Model file for the job. Use its own axes, mm. A direction names the side the tool comes from. Round coordinates to 2 decimals unless told otherwise and drop trailing zeros. Order: outer loops, then holes, each group sorted by start corner. A loop starts at its lowest first (then second) coordinate and runs counter-clockwise, first axis right, second up. Notation, with made-up numbers: (47.25, 61) - (87.25, 61) arc R11 cw to (87.25, 73) - close; hole circle Ø5 at (37, -26). An arc over 180 degrees is marked (long way). Put each result on its own line as item: value. Start each with the question number.
Item 1: Saw through at D-D on x = 8.5. List the corners of the cut face in (y, z), plus the area to 3 significant figures.
Item 2: Saw through at A-A on z = 9.25. List the corners of the cut face in (x, y).
Item 3: Saw through at C-C on z = -2. List the corners of the cut face in (x, y).
Item 4: Mould opens along X. For faces 4 (the face through (-11, 0, 1)), 5 (the face through (4, 0, 11.15)), 6 (the face through (0, 3, 2)) say: pulls with the +X half, pulls with the -X half, needs draft (parallel to the pull), parting line crosses it, or undercut.
Item 5: Saw through at B-B on y = -0.7. State how many separate pieces and enclosed holes the cut face has, plus the area to 3 significant figures.
Item 6: Which spindle directions (+Z, -Z, +X, -X, +Y, -Y) get a long thin tool onto all of the face, cutting with end or side? Do faces 1 (the face through (-6.1, 0, 7)), 2 (the face through (-1.984, 1, 7)), 3 (the face through (6.1, 0, 7)). Say none if no direction does.
Item 7: Probe probe 1 along X at (y, z) = (-1.5, 4.5); probe 2 along X at (y, z) = (1.3, -7.75); probe 3 along Z at (x, y) = (4, 1.45). List the from-to ranges inside material, lowest first.
Item 8: Pin check, flat tips, straight feed: pin 1 Ø3 at (x, y) = (1, -1) entering from -Z; pin 2 Ø1.5 at (y, z) = (-1.5, -7.5) entering from -X; pin 3 Ø1 at (x, z) = (-3.5, -1.5) entering from -Y; pin 4 Ø0.6 at (y, z) = (0.5, 1) entering from +X. Stop position of each tip, or through.
```python
from build123d import *

# Parameters (mm, degrees)
BOSS_EXTRUDE1_DEPTH  = 2.7
SKETCH2_R            = 1.5
CUT_EXTRUDE1_DEPTH   = 3.7
SKETCH3_W            = 4.115625
SKETCH3_H            = 6
BOSS_EXTRUDE2_DEPTH  = 8.7
SKETCH4_W            = 12
SKETCH4_H            = 3
CUT_EXTRUDE2_DEPTH   = 2
CUT_EXTRUDE3_DEPTH   = 0.25
SKETCH6_W            = 0.3
SKETCH6_H            = 0.3
BOSS_EXTRUDE3_DEPTH  = 12
LPATTERN1_COUNT      = 2
LPATTERN1_PITCH      = 2.5
LPATTERN1_COUNT_DIR2 = 2
LPATTERN1_PITCH_DIR2 = 9
SKETCH7_W            = 6.98
SKETCH7_H            = 0.5
CUT_EXTRUDE4_DEPTH   = 1


with BuildPart() as part:
    # Sketch1 → Boss-Extrude1 (new body)
    with BuildSketch(Plane.XY):
        with BuildLine():
            Line((-8, 3), (8, 3))
            ThreePointArc((8, 3), (11, 0), (8, -3))
            Line((8, -3), (-8, -3))
            ThreePointArc((-8, -3), (-11, 0), (-8, 3))
        make_face()
    extrude(amount=BOSS_EXTRUDE1_DEPTH)

    # Sketch2 → Cut-Extrude1 (cut, through all)
    with BuildSketch(Plane.XY.offset(2.7)):
        with Locations((-8.5, 0)):
            Circle(SKETCH2_R)
        with Locations((8.5, 0)):
            Circle(SKETCH2_R)
    extrude(amount=-CUT_EXTRUDE1_DEPTH, mode=Mode.SUBTRACT)

    # Sketch3 → Boss-Extrude2 (add)
    with BuildSketch(Plane.XY.offset(2.7)):
        with Locations((-4.0421875, 0)):
            Rectangle(SKETCH3_W, SKETCH3_H)
        with Locations((4.0421875, 0)):
            Rectangle(SKETCH3_W, SKETCH3_H)
    extrude(amount=BOSS_EXTRUDE2_DEPTH)

    # Sketch4 → Cut-Extrude2 (cut)
    with BuildSketch(Plane(origin=(0, 0, 0), x_dir=(-1, 0, 0), z_dir=(0, 0, -1))):
        Rectangle(SKETCH4_W, SKETCH4_H)
    extrude(amount=-CUT_EXTRUDE2_DEPTH, mode=Mode.SUBTRACT)

    # Sketch5 → Cut-Extrude3 (cut)
    with BuildSketch(Plane.XY.offset(11.4)):
        Polygon((-2.334375, 0.25), (-1.984375, 0.25), (-1.984375, -0.25), (-2.334375, -0.25), (-2.334375, -2.6), (-5.75, -2.6), (-5.75, 2.6), (-2.334375, 2.6), align=None)
    cut_extrude3 = extrude(amount=-CUT_EXTRUDE3_DEPTH, mode=Mode.SUBTRACT)

    # Mirror1: Cut-Extrude3 across plane
    add(cut_extrude3.mirror(Plane(origin=(0, 0, 0), x_dir=(0, 0, 1), z_dir=(1, 0, 0))), mode=Mode.SUBTRACT)

    # Sketch6 → Boss-Extrude3 (add)
    with BuildSketch(Plane(origin=(0, 0, 2), x_dir=(-1, 0, 0), z_dir=(0, 0, -1))):
        with Locations((-4.5, 1.25)):
            Rectangle(SKETCH6_W, SKETCH6_H)
    boss_extrude3 = extrude(amount=BOSS_EXTRUDE3_DEPTH)

    # LPattern1: Boss-Extrude3 2 × 2
    with Locations(*[(-j * LPATTERN1_PITCH_DIR2, -i * LPATTERN1_PITCH, 0) for i in range(LPATTERN1_COUNT) for j in range(LPATTERN1_COUNT_DIR2) if (i, j) != (0, 0)]):
        add(boss_extrude3)

    # Sketch7 → Cut-Extrude4 (cut)
    with BuildSketch(Plane.ZY.offset(-1.984375)):
        with Locations((6.19, 0)):
            Rectangle(SKETCH7_W, SKETCH7_H)
    cut_extrude4 = extrude(amount=-CUT_EXTRUDE4_DEPTH, mode=Mode.SUBTRACT)

    # Mirror2: Cut-Extrude4 across plane
    add(cut_extrude4.mirror(Plane(origin=(0, 0, 0), x_dir=(0, 0, 1), z_dir=(1, 0, 0))), mode=Mode.SUBTRACT)


solid = part.part
```
Results found:
1. outline: (-2.96, 0) - (-1.5, 0) - (-1.5, 2.7) - (-2.96, 2.7) - close; (1.5, 0) - (2.96, 0) - (2.96, 2.7) - (1.5, 2.7) - close
1. area: 7.87 mm²
2. outline: (-6.1, -3) - (-1.98, -3) - (-1.98, -0.25) - (-2.98, -0.25) - (-2.98, 0.25) - (-1.98, 0.25) - (-1.98, 3) - (-6.1, 3) - close; (1.98, -3) - (6.1, -3) - (6.1, 3) - (1.98, 3) - (1.98, 0.25) - (2.98, 0.25) - (2.98, -0.25) - (1.98, -0.25) - close
3. outline: (-4.65, -1.4) - (-4.35, -1.4) - (-4.35, -1.1) - (-4.65, -1.1) - close; (-4.65, 1.1) - (-4.35, 1.1) - (-4.35, 1.4) - (-4.65, 1.4) - close; (4.35, -1.4) - (4.65, -1.4) - (4.65, -1.1) - (4.35, -1.1) - close; (4.35, 1.1) - (4.65, 1.1) - (4.65, 1.4) - (4.35, 1.4) - close
4. face 4: pulls with the -X half
4. face 5: undercut
4. face 6: needs draft
5. separate pieces: 3
5. enclosed holes: 0
5. area: 90.5 mm²
6. face 1: +Z, -X, +Y, -Y
6. face 2: +Z, +Y, -Y
6. face 3: +Z, +X, +Y, -Y
7. probe 1: x = -6.1 to -1.98, 1.98 to 6.1
7. probe 2: x = -4.65 to -4.35, 4.35 to 4.65
7. probe 3: z = 2 to 11.15
8. pin 1: stops at z = 0
8. pin 2: stops at x = -4.65
8. pin 3: passes through
8. pin 4: stops at x = 10.99
